Job drawing, mm, ordinate dimensions from the low corner. One solid piece. Round coordinates to 2 decimals unless told otherwise and drop trailing zeros. Order: outer loops, then holes, each group sorted by start corner. A loop starts at its lowest first (then second) coordinate and runs counter-clockwise, first axis right, second up. Notation, with made-up numbers: (61.5, -22) -> (116.5, -22) arc R6 ccw to (116.5, -12) -> close; hole circle Ø5 at (89, -6). An arc over 180 degrees is marked (long way). Return JSON: item names as keys, results as strings. Group by question number.
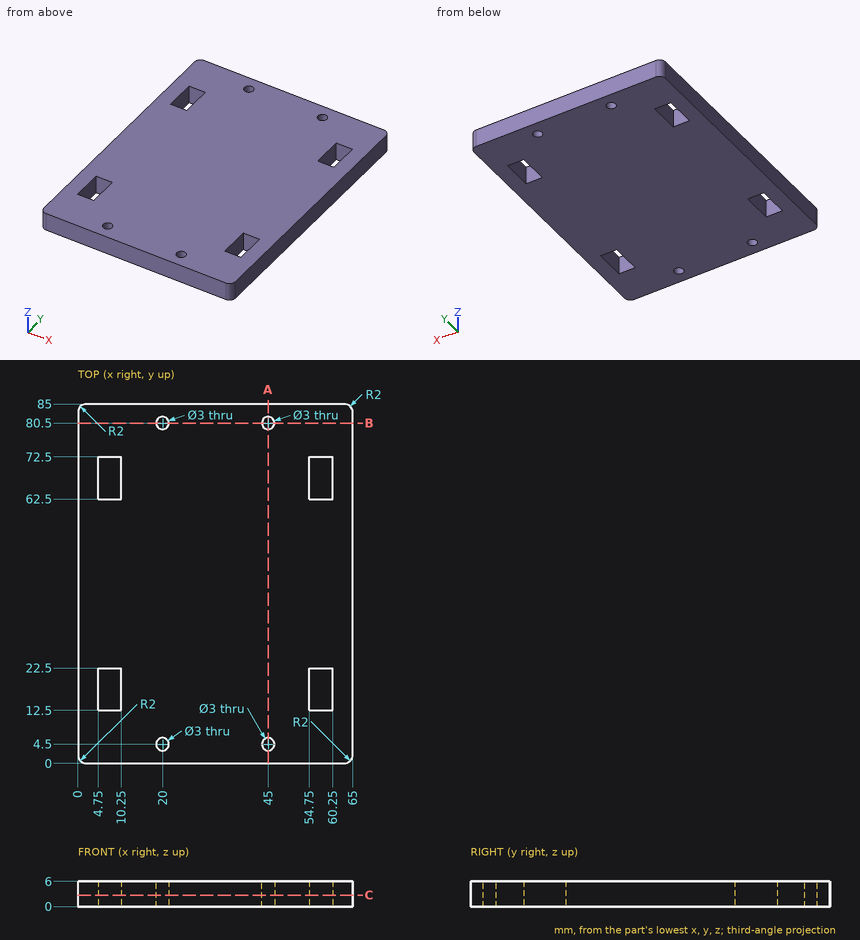
(1) Probe L1, parallel to Y at x = 20, z = 2.55; L2, parallel to Y at x = 5, z = 2.8; L3, parallel to X at y = 65, z = 1.85. List the from-to ranges inside material, lowest first. Write a range as [from, to].
(2) Saw through at A-A, the plane x = 45. List the corners of the cut face in (y, z), and give its area (3 significant figures).
(3) Saw through at C-C, the plane z = 2.7. State how many separate pieces and enclosed holes the cut face has, and give its area (3 significant figures).
(4) Saw through at B-B, the plane y = 80.5. List the corners of the cut face in (x, z).
Results are:
{
 "1": {"L1": "y = [0, 3], [6, 79], [82, 85]", "L2": "y = [0, 12.5], [22.5, 62.5], [72.5, 85]", "L3": "x = [0, 4.75], [10.25, 54.75], [60.25, 65]"},
 "2": {"outline": "(0, 0) -> (3, 0) -> (3, 6) -> (0, 6) -> close; (6, 0) -> (79, 0) -> (79, 6) -> (6, 6) -> close; (82, 0) -> (85, 0) -> (85, 6) -> (82, 6) -> close", "area": "474 mm^2"},
 "3": {"separate pieces": "1", "enclosed holes": "8", "area": "5,270 mm^2"},
 "4": {"outline": "(0, 0) -> (18.5, 0) -> (18.5, 6) -> (0, 6) -> close; (21.5, 0) -> (43.5, 0) -> (43.5, 6) -> (21.5, 6) -> close; (46.5, 0) -> (65, 0) -> (65, 6) -> (46.5, 6) -> close"}
}
